from build123d import *

# Parameters (mm, degrees)
F1_DEPTH = 2.54
F2_R     = 2.53999


# Not quite as in the source:
# - a fillet or chamfer is up to 0.001 mm smaller than in the source, because OpenCascade refuses the exact size


with BuildPart() as f1:
    # F0 (on Front) → F1 (new body, symmetric)
    with BuildSketch(Plane.XZ):
        with BuildLine():
            Line((-128.9416431369, 0), (-319.4416431369, 0))
            Line((-319.4416431369, 0), (-319.4416431369, -9.126868379))
            ThreePointArc((-319.4416431369, -9.126868379), (-224.2083966105, -11.8066385421), (-128.9416431369, -12.7))
            Line((-128.9416431369, -12.7), (-128.9416431369, 0))
        make_face()
        with BuildLine():
            Line((61.5583568631, 0), (-128.9416431369, 0))
            Line((-128.9416431369, 0), (-128.9416431369, -12.7))
            ThreePointArc((-128.9416431369, -12.7), (-33.6748896633, -11.8066385421), (61.5583568631, -9.126868379))
            Line((61.5583568631, -9.126868379), (61.5583568631, 0))
        make_face()
    extrude(amount=F1_DEPTH, both=True)

    # F2 (radius 2.54 in the source; OpenCascade refuses exactly that, so slightly less here)
    f2_edges = [f1.edges().sort_by_distance(p)[0] for p in [
        (-319.441643, -2.54, -4.563434),
        (-319.441643, 2.54, -4.563434),
        (61.558357, -2.54, -4.563434),
        (61.558357, 2.54, -4.563434),
    ]]
    fillet(f2_edges, radius=F2_R)


solid = f1.part
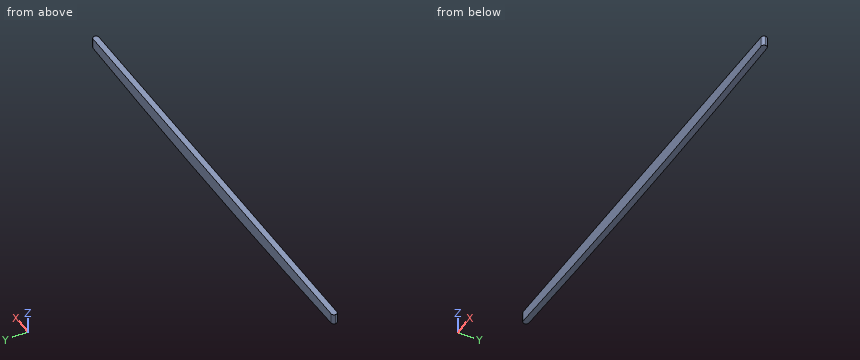
Can you work these out from the model? Positions are in its coordinate system, mm. Round coordinates to 2 decimals unless told otherwise and drop trailing zeros. Write each loop counter-clockwise with the first axis right and the second up, starting at its lowest first coordinate (ties: lowest second). Pieces come first, ordered by that corner, then holes. Notation, with made-up numbers: (72, 9) -> (129, 9) arc R22 ccw to (129, 32) -> close; hole circle Ø5 at (55.25, 61). An arc over 180 degrees is marked (long way). Use one line per item in the form item = value. Start each with the question number.
Q1. Imagine slicing it at B-B (y = 1.7). Please give me the cut outline in (x, z).
Q2. Imagine slicing it at A-A (x = 21). Please give me the cut outline in (y, z), then the cut area to 3 significant figures.
Q3. If I drill on probe 1 along X at (y, z) = (0.25, -2); probe 2 along X at (y, z) = (0.1, -5.75); probe 3 along Z at (x, y) = (11.5, 1.95), over which ranges is the centre line in solid material (lowest first)? Write a range as [from, to].
Worked out:
q1.outline = (-318.79, -9.15) arc R5080 ccw to (60.91, -9.15) -> (60.91, 0) -> (-318.79, 0) -> close
q2.outline = (-2.54, -10.49) -> (2.54, -10.49) -> (2.54, 0) -> (-2.54, 0) -> close
q2.area = 53.3 mm^2
q3.probe_1 = [-319.43, 61.55]
q3.probe_2 = [-319.44, 61.56]
q3.probe_3 = [-10.76, 0]
